from build123d import *

# Parameters (mm, degrees)
F1_DEPTH = 1.8
F2_R     = 1.5
F3_R     = 2.5
F4_SCALE = 10


with BuildPart() as f1:
    # F0 (on Right) → F1 (new body)
    with BuildSketch(Plane.YZ):
        with BuildLine():
            Line((20.157673577, -25.612176564), (20.157673577, 27.1963820784))
            Line((20.157673577, 27.1963820784), (0.3993508334, 34.387823436))
            Line((0.3993508334, 34.387823436), (-3.5206237808, 23.6177816987))
            ThreePointArc((-3.5206237808, 23.6177816987), (0.0725196424, 3.3694774982), (-11.6, -13.5614642316))
            Line((-11.6, -13.5614642316), (-26.0658084777, -16.112176564))
            Line((-26.0658084777, -16.112176564), (-23.0658084777, -25.612176564))
            Line((-23.0658084777, -25.612176564), (20.157673577, -25.612176564))
        make_face()
    extrude(amount=-F1_DEPTH)

    # F2
    f2_edges = [f1.edges().sort_by_distance(p)[0] for p in [
        (-0.9, -26.065808, -16.112177),
        (-0.9, -23.065808, -25.612177),
    ]]
    fillet(f2_edges, radius=F2_R)

    # F3
    f3_edges = [f1.edges().sort_by_distance(p)[0] for p in [
        (-0.9, 0.399351, 34.387823),
    ]]
    fillet(f3_edges, radius=F3_R)


with BuildPart() as f1_1:
    # F4: moved
    add(f1.part.scale(F4_SCALE).moved(Location((0, -181.4190621927, 230.5095890756))))


solid = f1_1.part
For this review, take the finished solid that the model builds, in its own axes (mm). Round coordinates to 2 decimals unless told otherwise and drop trailing zeros. Loops run counter-clockwise (first coordinate to the right, second up) from the corner with the lowest first, then second, coordinate; pieces in that order, holes last. Notation, with made-up numbers: (-32.5, 88) - (23.5, 88) arc R30 ccw to (23.5, 122) - close; hole circle Ø6 at (18, 44.25). An arc over 180 degrees is marked (long way). Put each result on its own line as item: value. Start each with the question number.
1. Consider section A-A on x = -8.25. State the section outline as (y, z) points (1 decimal).
2. Consider section B-B on y = -109.5. State the section outline as (x, z) points.
3. Insertion check: P1, Ø12, axis at y = -207, z = 205, coming from the -X side; P2, Ø1.5, axis at x = -2, z = 436.5, coming from the -Y side; P3, Ø4, axis at x = -5.5, y = -43.5, coming from the +Z side; P4, Ø6, axis at x = -8, z = 39.5, coming from the -Y side. Each pin has a flat end and moves straight along its axis. Give the tip position at first contact, or say it passes through.
4. Consider section C-C on z = 315. State the section outline as (x, y) points.
5. For probe 1 along Z at (x, y) = (-5, -165); probe 2 along Y at (x, z) = (-10.5, 237.5); probe 3 along Y at (x, z) = (-2, 235), list the stretches that pass through material, from the lowest coordinate up. Write a range as [from, to].
6. Mouldability with a two-part tool opening along Z and no side actions: class faces 1 (the cylindrical face through (-8.874, -180.082, 267.094)), 2 (the flat face through (-8.874, -426.307, 19.448)), 3 (the flat face through (-9, 20.158, 235)), 4 (the flat face through (-8.87, -65.67, 533.71)) as +Z half, -Z half, draft (parallel to the pull), parting line (faces both ways), or undercut.
Result sheet:
1. outline: (-436.9, 53.1) - (-415.4, -15.1) arc R15 ccw to (-401.1, -25.6) - (20.2, -25.6) - (20.2, 502.5) - (-153.9, 565.8) arc R25 ccw to (-186, 550.9) - (-216.6, 466.7) arc R270.7 cw to (-297.4, 94.9) - (-425.2, 72.4) arc R15 ccw to start
2. outline: (-18, -25.61) - (0, -25.61) - (0, 549.66) - (-18, 549.66) - close
3. P1: x = -18
3. P2: y = -200.42
3. P3: z = 526.37
3. P4: y = -433.59
4. outline: (-18, -174.6) - (0, -174.6) - (0, 20.16) - (-18, 20.16) - close
5. probe 1: [-25.61, 567.22]
5. probe 2: [-187.94, 20.16]
5. probe 3: [-188.78, 20.16]
6. face 1: undercut
6. face 2: -Z half
6. face 3: draft
6. face 4: +Z half
